from build123d import *

# Parameters (mm, degrees)
F0_W      = 101.6
F0_H      = 101.6
F1_DEPTH  = 101.6
F2_W      = 50.8
F2_H      = 76.2
F3_DEPTH  = 76.2
F4_W      = 25.4
F4_H      = 76.2
F5_DEPTH  = 63.5
F7_DEPTH  = 25.4
F9_DEPTH  = 25.4
F10_W     = 25.4
F10_H     = 19.05
F11_DEPTH = 25.4


with BuildPart() as f1:
    # F0 (on Front) → F1 (new body)
    with BuildSketch(Plane.XZ):
        with Locations((3.801119, 6.039162)):
            Rectangle(F0_W, F0_H)
    extrude(amount=F1_DEPTH)

    # F2 (on face) → F3 (cut)
    with BuildSketch(Plane.XZ.offset(101.6)):
        with Locations((3.801119, 18.739162)):
            Rectangle(F2_W, F2_H)
    extrude(amount=-F3_DEPTH, mode=Mode.SUBTRACT)

    # F4 (on face) → F5 (cut)
    with BuildSketch(Plane.XZ.offset(101.6)):
        with Locations((41.901119, 18.739162)):
            Rectangle(F4_W, F4_H)
        with Locations((-34.298881, 18.739162)):
            Rectangle(F4_W, F4_H)
    extrude(amount=-F5_DEPTH, mode=Mode.SUBTRACT)

    # F6 (on face) → F7 (cut)
    with BuildSketch(Plane.XY.offset(-19.360838)):
        Polygon((29.201119, -101.6), (54.601119, -101.6), (54.601119, -76.2), align=None)
    extrude(amount=-F7_DEPTH, mode=Mode.SUBTRACT)

    # F8 (on face) → F9 (cut)
    with BuildSketch(Plane.XY.offset(-19.360838)):
        Polygon((-46.998881, -76.2), (-46.998881, -101.6), (-21.598881, -101.6), align=None)
    extrude(amount=-F9_DEPTH, mode=Mode.SUBTRACT)

    # F10 (on face) → F11 (cut)
    with BuildSketch(Plane.XY.offset(-19.360838)):
        with Locations((3.801119, -66.675)):
            Rectangle(F10_W, F10_H)
    extrude(amount=-F11_DEPTH, mode=Mode.SUBTRACT)


solid = f1.part
Design review of the part built by this model. Coordinates are the model's own, in mm. A direction names the side the tool comes from. Coordinates: 2 decimals unless noted, no trailing zeros. Write each loop counter-clockwise with the first axis right and the second up, starting at its lowest first coordinate (ties: lowest second). Pieces come first, ordered by that corner, then holes. Notation, with made-up numbers: (61, -29) -> (111, -29) arc R9 ccw to (111, -17) -> close; hole circle Ø6 at (59.5, -33.75). An arc over 180 degrees is marked (long way). Write each question's results on one line, items separated by ' | '. Start each with the question number.
(1) Take a section at B-B on y = -68. Write out the cut boundary in (x, z), and give its area (3 significant figures).
(2) The part is to be moulded in two halves that separate along Y. For faces 6 (the face through (-8.899, -67, -32)), 7 (the face through (3, 0, 7)), 8 (the face through (42.1, -88.7, -31.9)), 9 (the face through (54.601, -29, -6)), say which applies: pulls with the +Y half, pulls with the -Y half, needs draft (parallel to the pull), parting line crosses it, or undercut.
(3) Take a section at D-D on y = -36.5. Write out the cut boundary in (x, z), and give its area (3 significant figures).
(4) Take a section at C-C on z = -27.5. Write out the cut boundary in (x, y).
(5) Clearance check with flat-ended pins moving along their axes: P1, Ø2, axis at x = 40, z = 40, coming from the -Y side; P2, Ø4, axis at x = 22.5, y = -35.5, coming from the +Z side; P3, Ø5, axis at x = -18.5, z = 30, coming from the -Y side. State where each tip first meets the part, or that it passes through.
(6) Tool access review of faces 1 (the face through (-46.999, -29, -6)), 2 (the face through (3, -25.4, 19)), 3 (the face through (-34.1, -89.1, -31.9)), 4 (the face through (-34, -38.1, 19)), 5 (the face through (16.501, -67, -32)): name each direction out of +Z, -Z, +X, -X, +Y, -Y from which nothing blocks a thin tool from reaching the whole face with its end or side.
(7) For line 1 along X through (y, z) = (-26.5, -0.5); line 2 along X through (y, z) = (-68, -33.5); line 3 along Y through (x, z) = (14, 25), list the stretches that pass through material, from the lowest coordinate up. Write a range as from..to.
(8) Take a section at A-A on x = 0.5. Write out the cut boundary in (y, z), and give its area (3 significant figures).
Results found:
1) outline: (-47, -44.76) -> (-8.9, -44.76) -> (-8.9, -19.36) -> (-47, -19.36) -> close; (16.5, -44.76) -> (54.6, -44.76) -> (54.6, -19.36) -> (16.5, -19.36) -> close | area: 1,940 mm2
2) face 6: undercut | face 7: pulls with the +Y half | face 8: pulls with the -Y half | face 9: needs draft
3) outline: (-47, -44.76) -> (54.6, -44.76) -> (54.6, 56.84) -> (29.2, 56.84) -> (29.2, -19.36) -> (-21.6, -19.36) -> (-21.6, 56.84) -> (-47, 56.84) -> close | area: 6,450 mm2
4) outline: (-47, -76.2) -> (-21.6, -101.6) -> (29.2, -101.6) -> (54.6, -76.2) -> (54.6, 0) -> (-47, 0) -> close; hole (-8.9, -76.2) -> (16.5, -76.2) -> (16.5, -57.15) -> (-8.9, -57.15) -> close
5) P1: stops at y = -38.1 | P2: stops at z = -19.36 | P3: stops at y = -25.4
6) face 1: +Z, -Z, -X, +Y, -Y | face 2: +Z, -Y | face 3: +Z, -Z, -X, -Y | face 4: +Z, +X, -X, -Y | face 5: +Z, -Z
7) line 1: x = -47..-21.6, 29.2..54.6 | line 2: x = -47..-8.9, 16.5..54.6 | line 3: y = -25.4..0
8) outline: (-101.6, -44.76) -> (-76.2, -44.76) -> (-76.2, -19.36) -> (-101.6, -19.36) -> close; (-57.15, -44.76) -> (0, -44.76) -> (0, 56.84) -> (-25.4, 56.84) -> (-25.4, -19.36) -> (-57.15, -19.36) -> close | area: 4,030 mm2
